from build123d import *

# Parameters (mm, degrees)
BOSS_EXTRUDE1_DEPTH = 1.5875
HOLE1_D             = 25.4


with BuildPart() as part:
    # Sketch2 → Boss-Extrude1 (new, symmetric)
    with BuildSketch(Plane(origin=(0, 0, 0), x_dir=(1, 0, 0), z_dir=(0, 1, 0))):
        with BuildLine():
            Line((20.6502, 3.302), (25.184455444, 3.302))
            ThreePointArc((25.184455444, 3.302), (17.960512242, 17.960512242), (3.302, 25.184455444))
            Line((3.302, 25.184455444), (3.302, 20.6502))
            ThreePointArc((3.302, 20.6502), (0, 17.3482), (-3.302, 20.6502))
            Line((-3.302, 20.6502), (-3.302, 25.184455444))
            ThreePointArc((-3.302, 25.184455444), (-17.960512242, 17.960512242), (-25.184455444, 3.302))
            Line((-25.184455444, 3.302), (-20.6502, 3.302))
            ThreePointArc((-20.6502, 3.302), (-17.3482, 0), (-20.6502, -3.302))
            Line((-20.6502, -3.302), (-25.184455444, -3.302))
            ThreePointArc((-25.184455444, -3.302), (-17.960512242, -17.960512242), (-3.302, -25.184455444))
            Line((-3.302, -25.184455444), (-3.302, -20.6502))
            ThreePointArc((-3.302, -20.6502), (0, -17.3482), (3.302, -20.6502))
            Line((3.302, -20.6502), (3.302, -25.184455444))
            ThreePointArc((3.302, -25.184455444), (17.960512242, -17.960512242), (25.184455444, -3.302))
            Line((25.184455444, -3.302), (20.6502, -3.302))
            ThreePointArc((20.6502, -3.302), (17.3482, 0), (20.6502, 3.302))
        make_face()
    extrude(amount=BOSS_EXTRUDE1_DEPTH, both=True)

    # Hole1 (through all)
    with Locations(Plane(origin=(0, 1.5875, 0), x_dir=(1, 0, 0), z_dir=(0, 1, 0))):
        with Locations((0, 0)):
            Hole(HOLE1_D / 2)


solid = part.part
Source: CAD feature listing. Evaluate the final solid. Frame: model axes, mm. A direction names the side the tool comes from. Round coordinates to 2 decimals unless told otherwise and drop trailing zeros. Order: outer loops, then holes, each group sorted by start corner. A loop starts at its lowest first (then second) coordinate and runs counter-clockwise, first axis right, second up. Notation, with made-up numbers: (-37.5, 57.25) - (-7.5, 57.25) arc R29 cw to (-7.5, 81.25) - close; hole circle Ø5 at (71, 82.5). An arc over 180 degrees is marked (long way). Use a Markdown table: item, result. Add a question column.
1. Section query C-C (x = 0). Return the cut outline in (y, z), then the cut area to 3 significant figures.
2. Line query: probe 1 along Z at (x, y) = (0, 0.8); probe 2 along X at (y, z) = (0.2, 22); probe 3 along X at (y, z) = (0.75, -10). Output: solid intervals per line, ascending.
3. Section query A-A (z = 0). Return the cut outline in (x, y).
4. Section query B-B (y = 1.05). Return the cut outline in (x, z).
5. First-contact query: pin 1 (1.6 mm diameter, centred on y = 0, z = -23.5, fed in from +X); pin 2 (1 mm diameter, centred on x = 23, y = -0.5, fed in from +Z); pin 3 (1 mm diameter, centred on y = 0.5, z = 23.5, fed in from +X). Flat tips, straight axial feed; report the tip coordinate or a pass-through.
6. Mould query, pull axis Z, two halves, no side actions, for faces 5 (the flat face through (-23, 0, 3.302)), 6 (the cylindrical face through (-0.07, 0.02, 17.35)), 7 (the cylindrical face through (-17.8, 0.02, -18.12)). Classes: +Z half, -Z half, draft (parallel to the pull), parting line (faces both ways), or undercut.
7. Set-up query: faces 1 (the flat face through (3.302, 0, 23)), 2 (the flat face through (23, 0, -3.302)), 3 (the flat face through (-23, 0, -3.302)), 4 (the flat face through (-3.302, 0, -23)). Return all of +Z, -Z, +X, -X, +Y, -Y with unobstructed straight access to the full face (end or side cutting, diameter ignored); none if empty.
Derived:
| question | item | result |
|---|---|---|
| 1 | outline | (-1.59, -17.35) - (1.59, -17.35) - (1.59, -12.7) - (-1.59, -12.7) - close; (-1.59, 12.7) - (1.59, 12.7) - (1.59, 17.35) - (-1.59, 17.35) - close |
| 1 | area | 29.5 mm2 |
| 2 | probe 1 | -17.35 to -12.7, 12.7 to 17.35 |
| 2 | probe 2 | -12.69 to -3.3, 3.3 to 12.69 |
| 2 | probe 3 | -23.35 to -7.83, 7.83 to 23.35 |
| 3 | outline | (-17.35, -1.59) - (-12.7, -1.59) - (-12.7, 1.59) - (-17.35, 1.59) - close; (12.7, -1.59) - (17.35, -1.59) - (17.35, 1.59) - (12.7, 1.59) - close |
| 4 | outline | (-25.18, -3.3) arc R25.4 ccw to (-3.3, -25.18) - (-3.3, -20.65) arc R3.3 cw to (3.3, -20.65) - (3.3, -25.18) arc R25.4 ccw to (25.18, -3.3) - (20.65, -3.3) arc R3.3 cw to (20.65, 3.3) - (25.18, 3.3) arc R25.4 ccw to (3.3, 25.18) - (3.3, 20.65) arc R3.3 cw to (-3.3, 20.65) - (-3.3, 25.18) arc R25.4 ccw to (-25.18, 3.3) - (-20.65, 3.3) arc R3.3 cw to (-20.65, -3.3) - close; hole circle Ø25.4 at (0, 0) |
| 5 | pin 1 | x = 11.4 |
| 5 | pin 2 | z = 11.79 |
| 5 | pin 3 | x = 10.78 |
| 6 | face 5 | undercut |
| 6 | face 6 | +Z half |
| 6 | face 7 | -Z half |
| 7 | face 1 | +Z, +Y, -Y |
| 7 | face 2 | +X, +Y, -Y |
| 7 | face 3 | -X, +Y, -Y |
| 7 | face 4 | -Z, +Y, -Y |
